```python
from build123d import *

# Parameters (mm, degrees)
CORTE_REVOLU_O2_ANGLE = 10.5
PADR_OCIRCULAR1_COUNT = 22


with BuildPart() as part:
    # Esboço1 → Revolução1 (revolve)
    with BuildSketch(Plane.XY, mode=Mode.PRIVATE) as revolu_o1_sk:
        with BuildLine():
            Line((0, 22.225), (104.772830684, 22.225))
            Line((104.772830684, 22.225), (104.772830684, 65.884431945))
            Line((104.772830684, 65.884431945), (63.025432751, 135))
            Line((63.025432751, 135), (63.025432751, 59.2125))
            ThreePointArc((63.025432751, 59.2125), (60.096500563, 52.141432188), (53.025432751, 49.2125))
            Line((53.025432751, 49.2125), (3.175, 49.2125))
            Line((3.175, 49.2125), (0, 46.0375))
            Line((0, 46.0375), (0, 22.225))
        make_face()
    revolve(revolu_o1_sk.sketch.rotate(Axis((0, 0, 0), (1, 0, 0)), 90), axis=Axis((0, 0, 0), (1, 0, 0)))  # turned: the seam where the file's is

    # Esboço3 → Corte-Revolução2 (revolve, symmetric, cut)
    with BuildSketch(Plane(origin=(0, 0, 0), x_dir=(1, 0, 0), z_dir=(0, 1, 0))) as corte_revolu_o2_sk:
        Polygon((104.772830684, 51.34699923), (63.025432751, 97.712181836), (63.025432751, 135), (111.527529929, 60.313319884), align=None)
    corte_revolu_o2 = revolve(axis=Axis((0, 0, 0), (1, 0, 0)), revolution_arc=CORTE_REVOLU_O2_ANGLE / 2, mode=Mode.SUBTRACT)
    corte_revolu_o2 = corte_revolu_o2 + revolve(corte_revolu_o2_sk.sketch, axis=Axis((0, 0, 0), (-1, 0, 0)), revolution_arc=CORTE_REVOLU_O2_ANGLE / 2, mode=Mode.SUBTRACT)

    # PadrãoCircular1: Corte-Revolução2 ×22 about axis
    padr_ocircular1_axis = Axis((0, 0, 0), (1, 0, 0))
    for i in range(1, PADR_OCIRCULAR1_COUNT):
        add(corte_revolu_o2.rotate(padr_ocircular1_axis, i * 360 / PADR_OCIRCULAR1_COUNT), mode=Mode.SUBTRACT)

    # Esboço2 → Corte-Revolução1 (revolve, cut)
    with BuildSketch(Plane.XY, mode=Mode.PRIVATE) as corte_revolu_o1_sk:
        Polygon((104.905562781, 58.449755058), (98.905562781, 52.449755058), (98.905562781, 18.901389006), (104.905562781, 18.901389006), align=None)
    revolve(corte_revolu_o1_sk.sketch.rotate(Axis((104.772830684, 0, 0), (-1, 0, 0)), 270), axis=Axis((104.772830684, 0, 0), (-1, 0, 0)), mode=Mode.SUBTRACT)  # turned: the seam where the file's is


solid = part.part
```
Design review of the part built by this model. Coordinates are the model's own, in mm. A direction names the side the tool comes from. Coordinates: 2 decimals unless noted, no trailing zeros. Loops run counter-clockwise (first coordinate to the right, second up) from the corner with the lowest first, then second, coordinate; pieces in that order, holes last.
Q1. We need section D-D on x = 59. State the section outline as (y, z) points (3 decimals), and give its area (3 significant figures).
Reported:
outline: circle Ø102.387 at (0, 0); hole circle Ø44.45 at (0, 0)
area: 6,680 mm2
Q2. We need section A-A on y = 0. State the section outline as (x, z) points (1 decimal), and give its area (3 significant figures).
Reported:
outline: (0, -46) - (3.2, -49.2) - (53, -49.2) arc R10 cw to (63, -59.2) - (63, -97.7) - (101.5, -55) - (98.9, -52.4) - (98.9, -22.2) - (0, -22.2) - close; (0, 22.2) - (98.9, 22.2) - (98.9, 52.4) - (101.5, 55) - (63, 97.7) - (63, 59.2) arc R10 cw to (53, 49.2) - (3.2, 49.2) - (0, 46) - close
area: 7,440 mm2
Q3. To check wall thickness, follow line 1 (Z direction, x = 92.5, y = 54.5); line 2 (Y direction, x = 24, z = 0) (1 decimal); line 3 (Y direction, x = 56.5, z = 0) (3 decimals). State the ranges of each line that lie inside material, in increasing order.
Reported:
line 1: z = -66.79 to -56.75, -39.1 to 39.1, 56.75 to 66.79
line 2: y = -49.2 to -22.2, 22.2 to 49.2
line 3: y = -49.836 to -22.225, 22.225 to 49.836
Q4. Tool access review of faces 4 (the face through (83.607, 41.992, 91.775)), 5 (the face through (80.9, 8.44, 91.84)), 6 (the face through (80.904, 92.111, 4.717)): name each direction out of +Z, -Z, +X, -X, +Y, -Y from which nothing blocks a thin tool from reaching the whole face with its end or side.
Reported:
face 4: +Z, +X, +Y
face 5: +Z, +X
face 6: +X
Q5. The part is to be moulded in two halves that separate along Y. For faces 1 (the face through (81.98, 58, 50.13)), 2 (the face through (80.9, 80.04, 45.83)), 3 (the face through (104.773, -41, 47)), say which applies: +Y half, -Y half, draft (parallel to the pull), parting line (faces both ways), or undercut.
Reported:
face 1: undercut
face 2: +Y half
face 3: draft
Q6. For pin 1 (5 mm diameter, centred on x = 30.5, z = 15, fed in from -Y); pin 2 (1.5 mm diameter, centred on x = 33.5, z = -36, fed in from -Y); pin 3 (5 mm diameter, centred on x = 89.5, y = -2, fed in from -Z), all flat-tipped, find the tip position at first contact; note any pin that passes through.
Reported:
pin 1: stops at y = -47.6
pin 2: stops at y = -34.34
pin 3: stops at z = -71.06
Q7. We need section C-C on y = -102. State how many separate pieces and enclosed holes the cut face has, and give its area (3 significant figures).
Reported:
separate pieces: 5
enclosed holes: 0
area: 843 mm2
